from build123d import *

# Parameters (mm, degrees)
F0_W     = 23
F0_H     = 15
F1_DEPTH = 8
F2_D     = 2
F2_DEPTH = 50
F3_D     = 10
F3_DEPTH = 50


with BuildPart() as f1:
    # F0 (on Top) → F1 (new body)
    with BuildSketch(Plane.XY):
        Rectangle(F0_W, F0_H)
        with BuildLine():
            Line((-11.5, -7.5), (-11.5, 7.5))
            ThreePointArc((-11.5, 7.5), (-32.024307, 2.863257), (-52.548613, 7.5))
            Line((-52.548613, 7.5), (-52.548613, 4))
            Line((-52.548613, 4), (-62.548613, 4))
            Line((-62.548613, 4), (-62.548613, 7.5))
            Line((-62.548613, 7.5), (-66.548613, 7.5))
            Line((-66.548613, 7.5), (-66.548613, -7.5))
            Line((-66.548613, -7.5), (-62.548613, -7.5))
            Line((-62.548613, -7.5), (-62.548613, -4))
            Line((-62.548613, -4), (-52.548613, -4))
            Line((-52.548613, -4), (-52.548613, -7.5))
            ThreePointArc((-52.548613, -7.5), (-32.024307, -2.863257), (-11.5, -7.5))
        make_face()
        with BuildLine():
            ThreePointArc((52.548613, 7.5), (32.024307, 2.863257), (11.5, 7.5))
            Line((11.5, 7.5), (11.5, -7.5))
            ThreePointArc((11.5, -7.5), (32.024307, -2.863257), (52.548613, -7.5))
            Line((52.548613, -7.5), (52.548613, -4))
            Line((52.548613, -4), (62.548613, -4))
            Line((62.548613, -4), (62.548613, -7.5))
            Line((62.548613, -7.5), (66.548613, -7.5))
            Line((66.548613, -7.5), (66.548613, 7.5))
            Line((66.548613, 7.5), (62.548613, 7.5))
            Line((62.548613, 7.5), (62.548613, 4))
            Line((62.548613, 4), (52.548613, 4))
            Line((52.548613, 4), (52.548613, 7.5))
        make_face()
    extrude(amount=F1_DEPTH)

    # F2
    with Locations(Plane(origin=(0, 0, 0), x_dir=(1, 0, 0), z_dir=(0, 0, -1))):
        with Locations((-57.820026, 1.5), (-57.820026, -1.5), (57.820026, 1.5), (57.820026, -1.5)):
            Hole(F2_D / 2, depth=F2_DEPTH)

    # F3
    with Locations(Plane(origin=(0, 0, 0), x_dir=(1, 0, 0), z_dir=(0, 0, -1))):
        with Locations((0, 0)):
            Hole(F3_D / 2, depth=F3_DEPTH)


solid = f1.part
Source: CAD feature listing. Evaluate the final solid. Frame: model axes, mm. A direction names the side the tool comes from. Round coordinates to 2 decimals unless told otherwise and drop trailing zeros. Loops run counter-clockwise (first coordinate to the right, second up) from the corner with the lowest first, then second, coordinate; pieces in that order, holes last. Notation, with made-up numbers: (31, 67.25) -> (55, 67.25) arc R18 ccw to (55, 86.25) -> close; hole circle Ø7 at (26, 13). An arc over 180 degrees is marked (long way). Answer as a JSON object with one key per item and string values. Group by question number.
Q1. Ray query, line 1 (Y direction, x = 0, z = 2.5); line 2 (X direction, y = 6.5, z = 0.75); line 3 (Y direction, x = -3, z = 5). Return the intervals inside material, ascending. Write a range as from..to.
Q2. Section query C-C (x = -43.5). Output: boundary loops of the cut face in (y, z), plus the area to 3 significant figures.
Q3. Access query for faces 4 (the flat face through (52.549, -6, 4)), 5 (the flat face through (52.549, 6, 4)), 6 (the flat face through (65, -7.5, 4)). Directions: +Z, -Z, +X, -X, +Y, -Y. A direction counts if a zero-diameter tool reaches every point of the face in a straight line with its end or side. Return the directions, or none.
Q4. Section query A-A (x = -3). Output: boundary loops of the cut face in (y, z).
Q5. Contact query for flat-ended pins moving along their axis: P1, Ø1, axis at x = 52.5, z = 6, coming from the -Y side; P2, Ø9, axis at x = 0, y = 0, coming from the -Z side; P3, Ø4, axis at x = -28, z = 6.5, coming from the -Y side; P4, Ø2.5, axis at x = -55, z = 4.5, coming from the -Y side. Output: stop coordinate, or through.
Q6. Section query D-D (x = 22). Output: boundary loops of the cut face in (y, z).
Q7. Mould query, pull axis X, two halves, no side actions, for faces 1 (the cylindrical face through (32.321, 2.864, 3.944)), 2 (the flat face through (66.549, 0, 4)), 3 (the flat face through (-65, -7.5, 4)). Classes: pulls with the +X half, pulls with the -X half, needs draft (parallel to the pull), parting line crosses it, or undercut.
Q8. Section query B-B (z = 4.5). State how many separate pieces and enclosed holes the cut face has, plus the area to 3 significant figures.
Completed:
{
 "1": {"line 1": "-7.5..-5, 5..7.5", "line 2": "-66.55..-62.55, -52.55..-50.3, -13.75..13.75, 50.3..52.55, 62.55..66.55", "line 3": "-7.5..-4, 4..7.5"},
 "2": {"outline": "(-4.26, 0) -> (4.26, 0) -> (4.26, 8) -> (-4.26, 8) -> close", "area": "68.2 mm²"},
 "3": {"face 4": "+Z, -Z, -Y", "face 5": "+Z, -Z, +Y", "face 6": "+Z, -Z, +X, -X, -Y"},
 "4": {"outline": "(-7.5, 0) -> (-4, 0) -> (-4, 8) -> (-7.5, 8) -> close; (4, 0) -> (7.5, 0) -> (7.5, 8) -> (4, 8) -> close"},
 "5": {"P1": "y = -7.5", "P2": "through", "P3": "y = -3.24", "P4": "y = -4"},
 "6": {"outline": "(-3.93, 0) -> (3.93, 0) -> (3.93, 8) -> (-3.93, 8) -> close"},
 "7": {"face 1": "undercut", "face 2": "pulls with the +X half", "face 3": "needs draft"},
 "8": {"separate pieces": "1", "enclosed holes": "5", "area": "1,250 mm²"}
}
